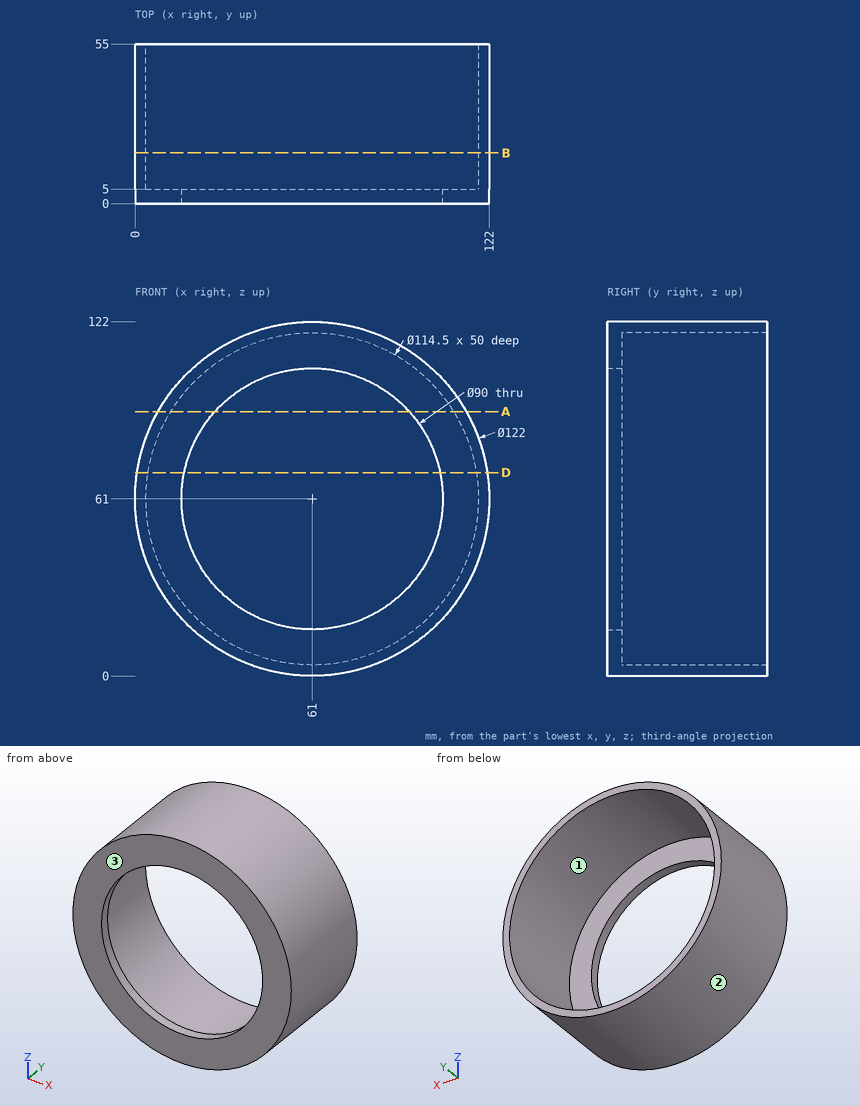
Answer from the drawing. Dimensions are ordinates in mm from the lowest x, y and z of the part. Coordinates: 2 decimals unless noted, no trailing zeros. Order: outer loops, then holes, each group sorted by start corner. A loop starts at its lowest first (then second) coordinate and runs counter-clockwise, first axis right, second up. Notation, with made-up numbers: M 21.5,-40 L 77.5,-40 A25 cw 77.5,-3 Z; hole C 46,55.25 d11. An arc over 180 degrees is marked long. Put each result on its own line as item: value. Start each with the question number.
Item 1: The mould has two halves that part along X. Classify the marked faces 1, 2 and 3: +X half, -X half, draft (parallel to the pull), parting line (faces both ways), or undercut.
Item 2: Consider probe 1 along Z at (x, y) = (60, 45.5); probe 2 along Z at (x, y) = (61, 2); probe 3 along X at (y, z) = (23.5, 54). Determine where each line is inside the solid, lowest interval first. Write a range as [from, to].
Item 3: Section D-D, the plane z = 70 is taken. Determine the outline of the cut face in (x, y).
Item 4: Given pin 1 Ø12 at (y, z) = (20, 83.5) entering from -X; pin 2 Ø1.5 at (x, y) = (80.5, 23) entering from +Z; pin 3 Ø12 at (y, z) = (48, 78.5) entering from +X, each flat-ended and moving along its own axis, determine where each tip first touches the part or whether it passes through.
Item 5: Section A-A, the plane z = 91 is taken. Determine the outline of the cut face in (x, y).
Item 6: Section B-B, the plane y = 17.5 is taken. Determine the outline of the cut face in (x, z).
Computed:
1. face 1: undercut
1. face 2: parting line
1. face 3: draft
2. probe 1: z = [0.01, 3.76], [118.24, 121.99]
2. probe 2: z = [0, 16], [106, 122]
2. probe 3: x = [0.4, 4.18], [117.82, 121.6]
3. outline: M 0.67,0 L 16.91,0 L 16.91,5 L 4.46,5 L 4.46,55 L 0.67,55 Z; M 105.09,0 L 121.33,0 L 121.33,55 L 117.54,55 L 117.54,5 L 105.09,5 Z
4. pin 1: stops at x = 2.27
4. pin 2: stops at z = 119.05
4. pin 3: stops at x = 120.91
5. outline: M 7.89,0 L 27.46,0 L 27.46,5 L 12.24,5 L 12.24,55 L 7.89,55 Z; M 94.54,0 L 114.11,0 L 114.11,55 L 109.76,55 L 109.76,5 L 94.54,5 Z
6. outline: C 61,61 d122; hole C 61,61 d114.5
